from build123d import *

# Parameters (mm, degrees)
PAD033_DEPTH    = 1
PAD034_DEPTH    = 17
POCKET020_DEPTH = 16
POCKET021_DEPTH = 11.6
SKETCH057_R     = 4
SKETCH057_R_2   = 1.95
SKETCH057_R_3   = 2
PAD035_DEPTH    = 5.5
SKETCH058_R     = 1.95
POCKET022_DEPTH = 8
POCKET023_DEPTH = 17


with BuildPart() as part:
    # Sketch053 → Pad033 (new body)
    with BuildSketch(Plane.XY):
        with BuildLine():
            Line((-49.75, 45), (-49.75, -45))
            ThreePointArc((-49.75, -45), (-49.457107, -45.707107), (-48.75, -46))
            Line((-48.75, -46), (48.75, -46))
            ThreePointArc((48.75, -46), (49.457107, -45.707107), (49.75, -45))
            Line((49.75, -45), (49.75, 45))
            ThreePointArc((49.75, 45), (49.457107, 45.707107), (48.75, 46))
            Line((48.75, 46), (-48.75, 46))
            ThreePointArc((-48.75, 46), (-49.457107, 45.707107), (-49.75, 45))
        make_face()
    extrude(amount=PAD033_DEPTH)

    # Sketch054 → Pad034 (join)
    with BuildSketch(Plane.XY):
        with BuildLine():
            Line((-49.75, 45), (-49.75, -45))
            ThreePointArc((-49.75, -45), (-49.457107, -45.707107), (-48.75, -46))
            Line((-48.75, -46), (48.75, -46))
            ThreePointArc((48.75, -46), (49.457107, -45.707107), (49.75, -45))
            Line((49.75, -45), (49.75, 45))
            ThreePointArc((49.75, 45), (49.457107, 45.707107), (48.75, 46))
            Line((48.75, 46), (-48.75, 46))
            ThreePointArc((-48.75, 46), (-49.457107, 45.707107), (-49.75, 45))
        make_face()
        Polygon((-47.75, 34), (-47.75, 21.8), (-8.75, 21.8), (-8.75, -38), (47.75, -38), (47.75, 34), align=None, mode=Mode.SUBTRACT)
    extrude(amount=PAD034_DEPTH)

    # Sketch055 (on Face14 of Pad034) → Pocket020 (cut)
    with BuildSketch(Plane.XY.offset(17)):
        with BuildLine():
            Line((-48.75, 45), (-48.75, 44))
            Line((-48.75, 44), (-10, 44))
            ThreePointArc((-8.5, 42.5), (-8.93934, 43.56066), (-10, 44))
            Line((-8.5, 42.5), (-8.5, 34))
            Line((-8.5, 34), (-7, 34))
            Line((-7, 34), (-7, 42.5))
            ThreePointArc((-5.5, 44), (-6.56066, 43.56066), (-7, 42.5))
            Line((-5.5, 44), (33.25, 44))
            Line((33.25, 44), (33.25, 37.5))
            Line((33.25, 37.5), (40.25, 37.5))
            Line((40.25, 37.5), (40.25, 34))
            Line((41.75, 34), (40.25, 34))
            Line((41.75, 37.5), (41.75, 34))
            Line((41.75, 37.5), (46.25, 37.5))
            Line((46.25, 37.5), (46.25, 34))
            Line((46.25, 34), (48.75, 34))
            Line((48.75, 45), (48.75, 34))
            Line((48.75, 45), (-48.75, 45))
        make_face()
    extrude(amount=-POCKET020_DEPTH, mode=Mode.SUBTRACT)

    # Sketch056 (on Face14 of Pocket020) → Pocket021 (cut)
    with BuildSketch(Plane.XY.offset(17)):
        Polygon((-11.794, 18.358), (-47.75, 18.358), (-47.75, -38), (-11.794, -38), (-11.794, -33), (-8.75, -33), (-8.75, 13.358), (-11.794, 13.358), align=None)
    extrude(amount=-POCKET021_DEPTH, mode=Mode.SUBTRACT)

    # Sketch057 → Pad035 (join)
    with BuildSketch(Plane.XY):
        with Locations((37.75, -6)):
            Circle(SKETCH057_R)
        with Locations((37.75, -6)):
            Circle(SKETCH057_R_2, mode=Mode.SUBTRACT)
        with Locations((37.75, -28)):
            Circle(SKETCH057_R)
        with Locations((37.75, -28)):
            Circle(SKETCH057_R_2, mode=Mode.SUBTRACT)
        with Locations((6.75, -17)):
            Circle(SKETCH057_R_3)
    extrude(amount=PAD035_DEPTH)

    # Sketch058 (on Face14 of Pad035) → Pocket022 (cut)
    with BuildSketch(Plane.XY.offset(17)):
        with Locations((-45.75, -42)):
            Circle(SKETCH058_R)
        with Locations((-30, -42)):
            Circle(SKETCH058_R)
        with Locations((30, -42)):
            Circle(SKETCH058_R)
        with Locations((-45.75, 40)):
            Circle(SKETCH058_R)
        with Locations((-30, 40)):
            Circle(SKETCH058_R)
        with Locations((30, 40)):
            Circle(SKETCH058_R)
        with Locations((45.75, -42)):
            Circle(SKETCH058_R)
    extrude(amount=-POCKET022_DEPTH, mode=Mode.SUBTRACT)

    # Sketch060 → Pocket023 (cut)
    with BuildSketch(Plane.XY):
        with BuildLine():
            ThreePointArc((-10, 0.5), (-15, -4.5), (-10, -9.5))
            Line((-10, -9.5), (10, -9.5))
            ThreePointArc((10, -9.5), (15, -4.5), (10, 0.5))
            Line((-10, 0.5), (10, 0.5))
        make_face()
    extrude(amount=POCKET023_DEPTH, mode=Mode.SUBTRACT)


solid = part.part
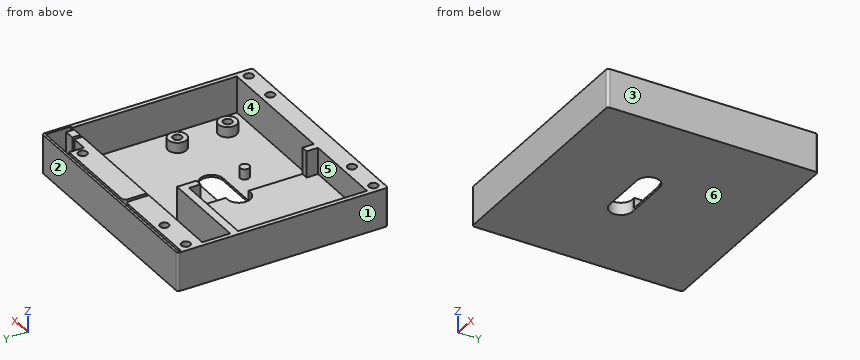
Could you check a few things on this model? Use its own coordinates, in mm. Face numbers are marked on the shaded views. A direction names the side the tool comes from. Give positions to 0.01 mm unless a question says otherwise; leave off trailing zeros. Order: outer loops, then holes, each group sorted by start corner. A loop starts at its lowest first (then second) coordinate and runs counter-clockwise, first axis right, second up.
1. We'd pull the mould along X, two halves only. Please class the marked faces 1, 2, 3 and 4: pulls with the +X half, pulls with the -X half, needs draft (parallel to the pull), parting line crosses it, or undercut.
2. Suppose I cut it at A-A (x = 30). List the corners of the cut face in (y, z) for me, plus the area to 3 significant figures.
3. For the marked faces 5 and 6, which set-ups out of +Z, -Z, +X, -X, +Y, -Y let a thin tool reach every point of the face, with its end or its side?
4. Suppose I cut it at B-B (y = 26). List the corners of the cut face in (x, z) for me.
5. Suppose I cut it at C-C (x = 6.5). List the corners of the cut face in (y, z) for me.
6. Will these pins go through, and if not, where does the flat tip stop? P1, Ø3, axis at x = 38, y = -7, coming from the +Z side; P2, Ø2, axis at x = -46, y = 40, coming from the +Z side; P3, Ø5, axis at x = 30.5, y = 6, coming from the +Z side.
7. Suppose I cut it at D-D (y = -6). List the corners of the cut face in (x, z) for me.
8. I need wall thicknesses on L1, parallel to Y at x = -14.5, z = 5.75; L2, parallel to Y at x = 30, z = 14.75; L3, parallel to Y at x = -30, z = 11. Which ranges of each line are inside material? Lowest first, please.
Solved:
1. face 1: pulls with the -X half
1. face 2: needs draft
1. face 3: pulls with the +X half
1. face 4: undercut
2. outline: (-46, 0) - (46, 0) - (46, 17) - (45, 17) - (45, 1) - (44, 1) - (44, 17) - (41.95, 17) - (41.95, 9) - (38.05, 9) - (38.05, 17) - (34, 17) - (34, 1) - (-38, 1) - (-38, 17) - (-40.05, 17) - (-40.05, 9) - (-43.95, 9) - (-43.95, 17) - (-46, 17) - close
2. area: 334 mm2
3. face 5: +Z
3. face 6: -Z, +X, -X, +Y, -Y
4. outline: (-49.75, 0) - (49.75, 0) - (49.75, 17) - (47.75, 17) - (47.75, 1) - (-47.75, 1) - (-47.75, 17) - (-49.75, 17) - close
5. outline: (-46, 0) - (-9.5, 0) - (-9.5, 1) - (-15.02, 1) - (-15.02, 5.5) - (-18.98, 5.5) - (-18.98, 1) - (-38, 1) - (-38, 17) - (-46, 17) - close; (0.5, 0) - (46, 0) - (46, 17) - (45, 17) - (45, 1) - (44, 1) - (44, 17) - (34, 17) - (34, 1) - (0.5, 1) - close
6. P1: stops at z = 5.5
6. P2: stops at z = 9
6. P3: stops at z = 1
7. outline: (-49.75, 0) - (-14.77, 0) - (-14.77, 5.4) - (-47.75, 5.4) - (-47.75, 17) - (-49.75, 17) - close; (14.77, 0) - (49.75, 0) - (49.75, 17) - (47.75, 17) - (47.75, 1) - (41.75, 1) - (41.75, 5.5) - (39.7, 5.5) - (39.7, 1) - (35.8, 1) - (35.8, 5.5) - (33.75, 5.5) - (33.75, 1) - (14.77, 1) - close
8. L1: y = -46 to -38, 18.36 to 21.8, 34 to 44, 45 to 46
8. L2: y = -46 to -43.95, -40.05 to -38, 34 to 38.05, 41.95 to 44, 45 to 46
8. L3: y = -46 to -43.95, -40.05 to -38, 18.36 to 21.8, 34 to 38.05, 41.95 to 44, 45 to 46
